```python
from build123d import *

# Parameters (mm, degrees)
F0_W     = 75
F0_H     = 31
F1_DEPTH = 3.81


with BuildPart() as f1:
    # F0 (on Top) → F1 (new body)
    with BuildSketch(Plane.XY):
        Polygon((62.5, 79), (62.5, 89), (-37.5, 89), (-37.5, 85.19), (-52.5, 85.19), (-52.5, 89), (-62.5, 89), (-62.5, 77), (-58.69, 77), (-58.69, 62), (-62.5, 62), (-62.5, 49.5), (-58.69, 49.5), (-58.69, 34.5), (-62.5, 34.5), (-62.5, 22.5), (-38.5, 22.5), (-38.5, 0), (-38.5, -22.5), (-62.5, -22.5), (-62.5, -34.5), (-58.69, -34.5), (-58.69, -49.5), (-62.5, -49.5), (-62.5, -62), (-58.69, -62), (-58.69, -77), (-62.5, -77), (-62.5, -89), (-52.5, -89), (-52.5, -85.19), (-37.5, -85.19), (-37.5, -89), (62.5, -89), (62.5, -79), (58.69, -79), (58.69, -64), (62.5, -64), (62.5, -54), (58.69, -54), (58.69, -39), (62.5, -39), (62.5, 39), (58.69, 39), (58.69, 54), (62.5, 54), (62.5, 64), (58.69, 64), (58.69, 79), align=None)
        with Locations((4, -65.5)):
            Rectangle(F0_W, F0_H, mode=Mode.SUBTRACT)
        with Locations((4, 65.5)):
            Rectangle(F0_W, F0_H, mode=Mode.SUBTRACT)
        Polygon((-38.5, 22.5), (-62.5, 22.5), (-62.5, -22.5), (-38.5, -22.5), (-38.5, 0), align=None)
    extrude(amount=F1_DEPTH)


solid = f1.part
```
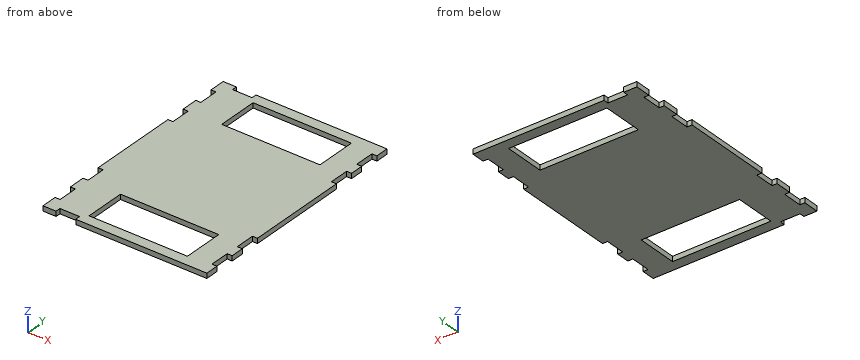
The model under review builds one solid part; all positions refer to its coordinate system, in mm. Round coordinates to 2 decimals unless told otherwise and drop trailing zeros. Write each loop counter-clockwise with the first axis right and the second up, starting at its lowest first coordinate (ties: lowest second). Pieces come first, ordered by that corner, then holes. Notation, with made-up numbers: (24.25, 87.5) - (42.25, 87.5) arc R16 cw to (42.25, 102.5) - close; hole circle Ø6 at (3, 13). An arc over 180 degrees is marked (long way). Answer as CSV lines item,"result". Start each with the question number.
(1) We need section D-D on y = 44. State the section outline as (x, z) points.
(2) For pin 1 Ø1.1 at (y, z) = (-69, 2.5) entering from +X; pin 2 Ø1.1 at (y, z) = (-67.5, 1.5) entering from -X, all flat-tipped, find the tip position at first contact; note any pin that passes through.
(3) We need section A-A on x = -8. State the section outline as (y, z) points, plus the area to 3 significant figures.
(4) We need section B-B on z = 0.85. Give the number of separate pieces and of enclosed holes in the cut face, plus the area to 3 significant figures.
(5) We need section C-C on x = -45.5. State the section outline as (y, z) points.
(6) To check wall thickness, follow line 1 (Y direction, x = -7.5, z = 3.45); line 2 (X direction, y = -59, z = 2.3); line 3 (Y direction, x = -39, z = 0.75). State the ranges of each line that lie inside material, in increasing order.
Worked answers:
1,outline,"(-58.69, 0) - (58.69, 0) - (58.69, 3.81) - (-58.69, 3.81) - close"
2,pin 1,"x = 58.69"
2,pin 2,"x = -58.69"
3,outline,"(-89, 0) - (-81, 0) - (-81, 3.81) - (-89, 3.81) - close; (-50, 0) - (50, 0) - (50, 3.81) - (-50, 3.81) - close; (81, 0) - (89, 0) - (89, 3.81) - (81, 3.81) - close"
3,area,"442 mm²"
4,separate pieces,"1"
4,enclosed holes,"2"
4,area,"17,000 mm²"
5,outline,"(-85.19, 0) - (85.19, 0) - (85.19, 3.81) - (-85.19, 3.81) - close"
6,line 1,"-89 to -81, -50 to 50, 81 to 89"
6,line 2,"-62.5 to -33.5, 41.5 to 62.5"
6,line 3,"-85.19 to 85.19"
